from build123d import *

# Parameters (mm, degrees)
SKETCH002_W             = 119.3
SKETCH002_H             = 68.7
PAD001_DEPTH            = 3.6
SKETCH003_W             = 109.6
SKETCH003_H             = 61.6
PAD002_DEPTH            = 0.3
SKETCH004_W             = 26
SKETCH004_H             = 55.7
PAD003_DEPTH            = 1
SKETCH006_R             = 2.365045
PAD004_DEPTH            = 10
BODY001_PLACEMENT_ANGLE = 180


with BuildPart() as part:
    # Sketch002 → Pad001 (new body)
    with BuildSketch(Plane.XZ):
        Rectangle(SKETCH002_W, SKETCH002_H)
    extrude(amount=PAD001_DEPTH)

    # Sketch003 → Pad002 (join)
    with BuildSketch(Plane.XZ.offset(3.5)):
        with Locations((3.15, 0)):
            Rectangle(SKETCH003_W, SKETCH003_H)
    extrude(amount=PAD002_DEPTH)

    # Sketch004 → Pad003 (join)
    with BuildSketch(Plane.XZ.offset(-1)):
        with Locations((-46.65, -6.5)):
            Rectangle(SKETCH004_W, SKETCH004_H)
    extrude(amount=PAD003_DEPTH)

    # Sketch006 → Pad004 (join)
    with BuildSketch(Plane.XZ):
        with Locations((3.15, 0)):
            Circle(SKETCH006_R)
    extrude(amount=PAD004_DEPTH)


with BuildPart() as part_1:
    # Body001 placement: moved
    add(part.part.moved(Location((3, -5, 41))).rotate(Axis((3, -5, 41), (0, 1, 0)), BODY001_PLACEMENT_ANGLE))


solid = part_1.part
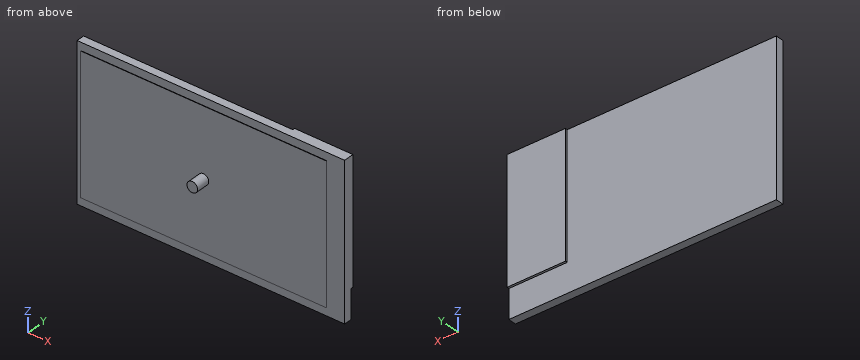
Here's how the part is built. I have some questions about the finished solid (model axes, mm). Coordinates: 2 decimals unless noted, no trailing zeros. Write each loop counter-clockwise with the first axis right and the second up, starting at its lowest first coordinate (ties: lowest second). Pieces come first, ordered by that corner, then holes.
Item 1: I want a section at D-D on z = 12. Write out the boundary of the cut face in (x, y), and give its area (3 significant figures).
Item 2: I want a section at C-C on x = -32.5. Write out the boundary of the cut face in (y, z).
Item 3: Will these pins go through, and if not, where does the flat tip stop? pin 1 (4 mm diameter, centred on x = -25.5, z = 14, fed in from -Y); pin 2 (4 mm diameter, centred on y = -11, z = 15, fed in from -X); pin 3 (0.8 mm diameter, centred on y = -4.5, z = 40, fed in from -X).
Item 4: If I drill on line 1 (Y direction, x = -34, z = 43.5); line 2 (Y direction, x = 55, z = 59.5); line 3 (X direction, y = -14.5, z = 42), over which ranges is the centre line in solid material (lowest first)?
Item 5: I want a section at B-B on z = 36. Write out the boundary of the cut face in (x, y), and give its area (3 significant figures).
Item 6: I want a section at A-A on x = -0.15. Write out the boundary of the cut face in (y, z).
Findings below:
1. outline: (-56.65, -8.6) - (-54.95, -8.6) - (-54.95, -8.8) - (54.65, -8.8) - (54.65, -8.6) - (62.65, -8.6) - (62.65, -5) - (-56.65, -5) - close
1. area: 451 mm2
2. outline: (-8.8, 10.2) - (-8.6, 10.2) - (-8.6, 6.65) - (-5, 6.65) - (-5, 75.35) - (-8.6, 75.35) - (-8.6, 71.8) - (-8.8, 71.8) - close
3. pin 1: stops at y = -8.8
3. pin 2: passes through
3. pin 3: stops at x = 36.65
4. line 1: y = -8.8 to -5
4. line 2: y = -8.6 to -4
4. line 3: x = -2.29 to 1.99
5. outline: (-56.65, -8.6) - (-54.95, -8.6) - (-54.95, -8.8) - (54.65, -8.8) - (54.65, -8.6) - (62.65, -8.6) - (62.65, -4) - (36.65, -4) - (36.65, -5) - (-56.65, -5) - close
5. area: 477 mm2
6. outline: (-15, 38.63) - (-8.8, 38.63) - (-8.8, 10.2) - (-8.6, 10.2) - (-8.6, 6.65) - (-5, 6.65) - (-5, 75.35) - (-8.6, 75.35) - (-8.6, 71.8) - (-8.8, 71.8) - (-8.8, 43.37) - (-15, 43.37) - close
